For this review, use the dimensioned drawing (mm, ordinates from the lowest corner) and the shaded views. Round coordinates to 2 decimals unless told otherwise and drop trailing zeros. Loops run counter-clockwise (first coordinate to the right, second up) from the corner with the lowest first, then second, coordinate; pieces in that order, holes last. Notation, with made-up numbers: (45, -1.5) - (81, -1.5) arc R27 ccw to (81, 21.5) - close; hole circle Ø3 at (-28.75, -30.75). An arc over 180 degrees is marked (long way). One line per question, with ' | ' between items. Start each with the question number.
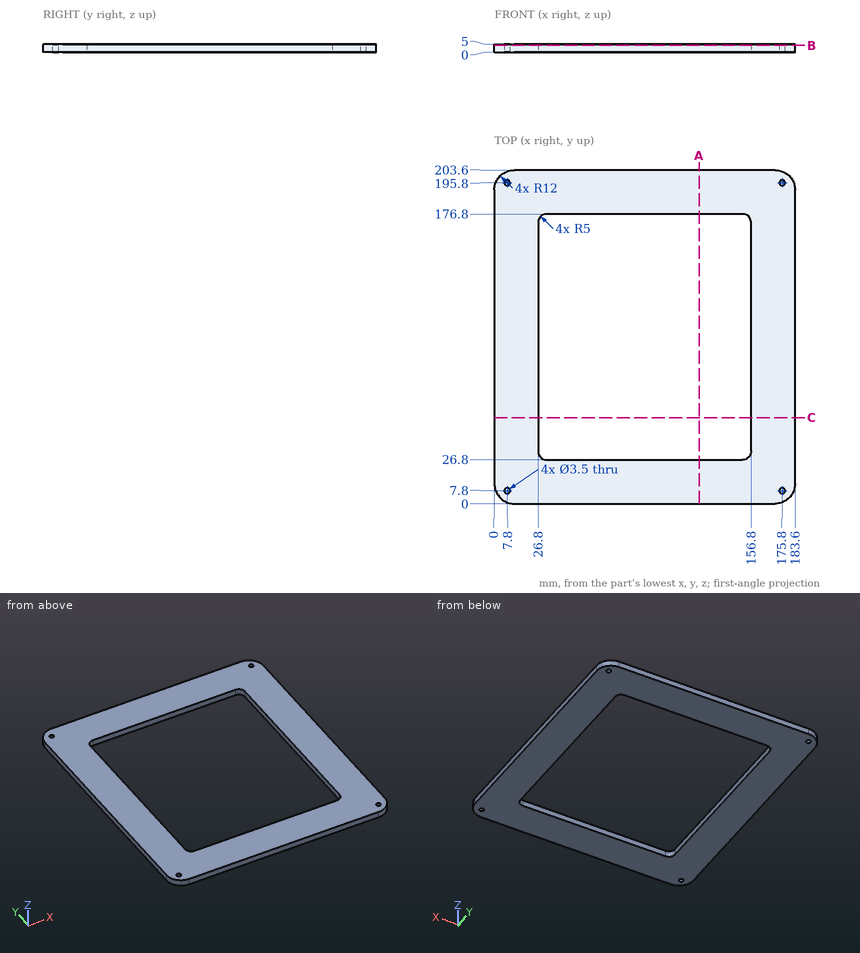
1. Take a section at B-B, the plane z = 4.1. Give the boundary of the cut face in (x, y).
2. To check wall thickness, follow line 1 along X through (y, z) = (121.5, 4.55); line 2 along Y through (x, z) = (88.5, 2.3); line 3 along X through (y, z) = (195.8, 3.6). State the ranges of each line that lie inside material, in increasing order.
3. Take a section at A-A, the plane x = 125. Give the boundary of the cut face in (y, z), then the cut area to 3 significant figures.
4. Take a section at C-C, the plane y = 52.5. Give the boundary of the cut face in (x, z), then the cut area to 3 significant figures.
Answer list:
1) outline: (0, 12) arc R12 ccw to (12, 0) - (171.6, 0) arc R12 ccw to (183.6, 12) - (183.6, 191.6) arc R12 ccw to (171.6, 203.6) - (12, 203.6) arc R12 ccw to (0, 191.6) - close; hole circle Ø3.5 at (7.8, 7.8); hole circle Ø3.5 at (7.8, 195.8); hole (26.8, 31.8) arc R5 ccw to (31.8, 26.8) - (151.8, 26.8) arc R5 ccw to (156.8, 31.8) - (156.8, 171.8) arc R5 ccw to (151.8, 176.8) - (31.8, 176.8) arc R5 ccw to (26.8, 171.8) - close; hole circle Ø3.5 at (175.8, 7.8); hole circle Ø3.5 at (175.8, 195.8)
2) line 1: x = 0 to 26.8, 156.8 to 183.6 | line 2: y = 0 to 26.8, 176.8 to 203.6 | line 3: x = 0.76 to 6.05, 9.55 to 174.05, 177.55 to 182.84
3) outline: (0, 0) - (26.8, 0) - (26.8, 5) - (0, 5) - close; (176.8, 0) - (203.6, 0) - (203.6, 5) - (176.8, 5) - close | area: 268 mm²
4) outline: (0, 0) - (26.8, 0) - (26.8, 5) - (0, 5) - close; (156.8, 0) - (183.6, 0) - (183.6, 5) - (156.8, 5) - close | area: 268 mm²
